from build123d import *

# Parameters (mm, degrees)
SKETCH_1_R          = 18.9
EXTRUDE_1_DEPTH     = 36.94
SKETCH_2_R          = 17.81
EXTRUDE_2_DEPTH     = 3.23
EXTRUDE_START       = 16.99
SKETCH_3_R          = 17.81
EXTRUDE_3_DEPTH     = 16.99
SKETCH_4_R          = 16.485
CUT_EXTRUDE_1_DEPTH = 1.38
SKETCH_5_R          = 12.15
EXTRUDE_4_DEPTH     = 1
SKETCH_6_R          = 5.125
EXTRUDE_5_DEPTH     = 4
SKETCH_7_R          = 4.49987444
CUT_EXTRUDE_2_DEPTH = 1
SKETCH_8_R          = 1.275207664
EXTRUDE_6_DEPTH     = 4
SKETCH_9_R          = 7.280511115
EXTRUDE_7_DEPTH     = 4
SKETCH_10_R         = 6.024089917
CUT_EXTRUDE_3_DEPTH = 2.5
SKETCH_11_R         = 1.805272954
EXTRUDE_9_DEPTH     = 10


with BuildPart() as part:
    # 草图1 → 凸台-拉伸1 (new body)
    with BuildSketch(Plane.XY):
        Circle(SKETCH_1_R)
    extrude(amount=EXTRUDE_1_DEPTH)

    # 草图2 → 凸台-拉伸2 (add)
    with BuildSketch(Plane.XY.offset(36.94)):
        Circle(SKETCH_2_R)
    extrude(amount=EXTRUDE_2_DEPTH)

    # 草图3 → 凸台-拉伸3 (add)
    with BuildSketch(Plane(origin=(0, 0, 0), x_dir=(-1, 0, 0), z_dir=(0, 0, -1)).offset(EXTRUDE_START)):
        with Locations(Location((0, 0, 0), (0, 0, 180))):
            Circle(SKETCH_3_R)
    extrude(amount=-EXTRUDE_3_DEPTH)

    # 草图4 → 切除-拉伸1 (cut)
    with BuildSketch(Plane(origin=(0, 0, -16.99), x_dir=(-1, 0, 0), z_dir=(0, 0, -1))):
        Circle(SKETCH_4_R)
    extrude(amount=-CUT_EXTRUDE_1_DEPTH, mode=Mode.SUBTRACT)

    # 草图5 → 凸台-拉伸4 (add)
    with BuildSketch(Plane(origin=(0, 0, -15.61), x_dir=(-1, 0, 0), z_dir=(0, 0, -1))):
        Circle(SKETCH_5_R)
    extrude(amount=EXTRUDE_4_DEPTH)

    # 草图6 → 凸台-拉伸5 (add)
    with BuildSketch(Plane(origin=(0, 0, -16.61), x_dir=(-1, 0, 0), z_dir=(0, 0, -1))):
        Circle(SKETCH_6_R)
    extrude(amount=EXTRUDE_5_DEPTH)

    # 草图7 → 切除-拉伸2 (cut)
    with BuildSketch(Plane(origin=(0, 0, -20.61), x_dir=(-1, 0, 0), z_dir=(0, 0, -1))):
        Circle(SKETCH_7_R)
    extrude(amount=-CUT_EXTRUDE_2_DEPTH, mode=Mode.SUBTRACT)

    # 草图8 → 凸台-拉伸6 (add)
    with BuildSketch(Plane(origin=(0, 0, -19.61), x_dir=(-1, 0, 0), z_dir=(0, 0, -1))):
        Circle(SKETCH_8_R)
    extrude(amount=EXTRUDE_6_DEPTH)

    # 草图9 → 凸台-拉伸7 (add)
    with BuildSketch(Plane.XY.offset(40.17)):
        Circle(SKETCH_9_R)
    extrude(amount=EXTRUDE_7_DEPTH)

    # 草图10 → 切除-拉伸3 (cut)
    with BuildSketch(Plane.XY.offset(44.17)):
        Circle(SKETCH_10_R)
    extrude(amount=-CUT_EXTRUDE_3_DEPTH, mode=Mode.SUBTRACT)

    # 草图11 → 凸台-拉伸9 (add)
    with BuildSketch(Plane.XY.offset(41.67)):
        Circle(SKETCH_11_R)
    extrude(amount=EXTRUDE_9_DEPTH)


solid = part.part
Geometry check sheet. Reference: the model listing, model coordinates, mm. A direction names the side the tool comes from. Round coordinates to 2 decimals unless told otherwise and drop trailing zeros. Order: outer loops, then holes, each group sorted by start corner. A loop starts at its lowest first (then second) coordinate and runs counter-clockwise, first axis right, second up. Notation, with made-up numbers: M -23,89.5 L 18,89.5 A16 ccw 18,114.5 Z; hole C 68.5,72.25 d4. An arc over 180 degrees is marked long. Answer in a Markdown table with one row per item. Add a question column.
Item 1: Sectioned sample at C-C, the plane y = 9. Enter the section's corners in (x, z).
Item 2: Depth check by flat-ended pin: pin 1 Ø12 at (x, y) = (12.5, -6.5) entering from +Z; pin 2 Ø12 at (y, z) = (-3, 43.5) entering from +X; pin 3 Ø12 at (x, z) = (-5, 8.5) entering from +Y. Enter the tip coordinate at first touch or a pass-through.
Item 3: Sectioned sample at D-D, the plane x = -8.5. Enter the section's corners in (y, z), plus the area to 3 significant figures.
Item 4: Draft check along X on faces 4 (the face through (-4.292, 1.352, -20.117)), 5 (the face through (-2, 6, 44.17)), 6 (the face through (-3.861, 17.386, -8.614)), 7 (the face through (5.746, 1.809, 42.938)). Enter one of: released by +X, released by -X, zero draft, split by the parting line, or undercut.
Item 5: Material ranges on L1, parallel to Y at x = 0, z = -20.1 (3 decimals); L2, parallel to Y at x = 0, z = -16.65 (3 decimals); L3, parallel to Z at x = 5, y = 16.5, recorded low to high. Write a range as [from, to].
Item 6: Sectioned sample at A-A, the plane x = -13. Enter the section's corners in (y, z), plus the area to 3 significant figures.
Item 7: Set-up check for faces 1 (the face through (-3.861, -17.386, 38.532)), 2 (the face through (1.111, -5.003, -18.582)), 3 (the face through (0, 0, 51.67)): record each of +Z, -Z, +X, -X, +Y, -Y from which the full face is reachable in a straight line by a thin tool's end or side.
Item 8: Sectioned sample at B-B, the plane z = 2.5. Enter the section's corners in (x, y), plus the area to 3 significant figures.
Filled in:
| question | item | result |
|---|---|---|
| 1 | outline | M -16.62,0 L -15.37,0 L -15.37,-16.99 L -13.81,-16.99 L -13.81,-15.61 L -8.16,-15.61 L -8.16,-16.61 L 8.16,-16.61 L 8.16,-15.61 L 13.81,-15.61 L 13.81,-16.99 L 15.37,-16.99 L 15.37,0 L 16.62,0 L 16.62,36.94 L 15.37,36.94 L 15.37,40.17 L -15.37,40.17 L -15.37,36.94 L -16.62,36.94 Z |
| 2 | pin 1 | stops at z = 40.17 |
| 2 | pin 2 | stops at x = 17.81 |
| 2 | pin 3 | stops at y = 18.9 |
| 3 | outline | M -16.88,0 L -15.65,0 L -15.65,-16.99 L -14.12,-16.99 L -14.12,-15.61 L -8.68,-15.61 L -8.68,-16.61 L 8.68,-16.61 L 8.68,-15.61 L 14.12,-15.61 L 14.12,-16.99 L 15.65,-16.99 L 15.65,0 L 16.88,0 L 16.88,36.94 L 15.65,36.94 L 15.65,40.17 L -15.65,40.17 L -15.65,36.94 L -16.88,36.94 Z |
| 3 | area | 1,860 mm² |
| 4 | face 4 | undercut |
| 4 | face 5 | zero draft |
| 4 | face 6 | split by the parting line |
| 4 | face 7 | undercut |
| 5 | L1 | y = [-5.125, -4.5], [-1.275, 1.275], [4.5, 5.125] |
| 5 | L2 | y = [-17.81, -16.485], [-5.125, 5.125], [16.485, 17.81] |
| 5 | L3 | z = [-16.99, 40.17] |
| 6 | outline | M -13.72,0 L -12.17,0 L -12.17,-16.99 L -10.14,-16.99 L -10.14,-15.61 L 10.14,-15.61 L 10.14,-16.99 L 12.17,-16.99 L 12.17,0 L 13.72,0 L 13.72,36.94 L 12.17,36.94 L 12.17,40.17 L -12.17,40.17 L -12.17,36.94 L -13.72,36.94 Z |
| 6 | area | 1,480 mm² |
| 7 | face 1 | +Z |
| 7 | face 2 | -Z |
| 7 | face 3 | +Z, +X, -X, +Y, -Y |
| 8 | outline | C 0,0 d37.8 |
| 8 | area | 1,120 mm² |
